Build history of the part. All positions in model axes, mm. A direction names the side the tool comes from. Coordinates: 2 decimals unless noted, no trailing zeros. Write each loop counter-clockwise with the first axis right and the second up, starting at its lowest first coordinate (ties: lowest second). Pieces come first, ordered by that corner, then holes.
```python
from build123d import *

# Parameters (mm, degrees)
SKETCH1_W                       = 149
SKETCH1_H                       = 40
SKETCH1_W_2                     = 6.3
SKETCH1_H_2                     = 6.3
BOSS_EXTRUDE1_DEPTH             = 12.7
TAP_DRILL_FOR_M5X0_8_TAP2_D     = 4.2
TAP_DRILL_FOR_M5X0_8_TAP2_DEPTH = 7
TAP_DRILL_FOR_M5X0_8_TAP2_TIP   = 1.2618073
TAP_DRILL_FOR_M5X0_8_TAP3_D     = 4.2


with BuildPart() as part:
    # Sketch1 → Boss-Extrude1 (new body)
    with BuildSketch(Plane.XY):
        with Locations((0, 20)):
            Rectangle(SKETCH1_W, SKETCH1_H)
        with Locations((35, 20)):
            Rectangle(SKETCH1_W_2, SKETCH1_H_2, mode=Mode.SUBTRACT)
    extrude(amount=BOSS_EXTRUDE1_DEPTH)

    # Tap Drill for M5x0.8 Tap2
    with Locations(Plane(origin=(-60, 0, 6.35), x_dir=(-1, 0, 0), z_dir=(0, -1, 0))):
        with Locations((0, 0), (-60, 0), (-120, 0)):
            Hole(TAP_DRILL_FOR_M5X0_8_TAP2_D / 2, depth=TAP_DRILL_FOR_M5X0_8_TAP2_DEPTH)
            with Locations((0, 0, -(TAP_DRILL_FOR_M5X0_8_TAP2_DEPTH + TAP_DRILL_FOR_M5X0_8_TAP2_TIP / 2))):  # 118° drill point
                Cone(0, TAP_DRILL_FOR_M5X0_8_TAP2_D / 2, TAP_DRILL_FOR_M5X0_8_TAP2_TIP, mode=Mode.SUBTRACT)

    # Tap Drill for M5x0.8 Tap3 (through all)
    with Locations(Plane.XY.offset(12.7)):
        with Locations((-65, 30), (-65, 10), (65, 10), (65, 30)):
            Hole(TAP_DRILL_FOR_M5X0_8_TAP3_D / 2)


solid = part.part
```
1. 3-axis set-ups, long thin cutter, end or side, ignore diameter. For faces 4 (the face through (-74.5, 20, 6)), 5 (the face through (-0.46, 3.55, 8.4)), 6 (the face through (35, 16.85, 6)): which of +Z, -Z, +X, -X, +Y, -Y reach the whole face in a straight line?
Computed values:
face 4: +Z, -Z, -X, +Y, -Y
face 5: -Y
face 6: +Z, -Z
2. Saw through at C-C on z = 11.25. List the corners of the cut face in (x, y).
Computed values:
outline: (-74.5, 0) - (74.5, 0) - (74.5, 40) - (-74.5, 40) - close; hole circle Ø4.2 at (-65, 10); hole circle Ø4.2 at (-65, 30); hole (31.85, 16.85) - (38.15, 16.85) - (38.15, 23.15) - (31.85, 23.15) - close; hole circle Ø4.2 at (65, 10); hole circle Ø4.2 at (65, 30)
3. Saw through at A-A on x = 65. List the corners of the cut face in (y, z).
Computed values:
outline: (0, 0) - (7.9, 0) - (7.9, 12.7) - (0, 12.7) - close; (12.1, 0) - (27.9, 0) - (27.9, 12.7) - (12.1, 12.7) - close; (32.1, 0) - (40, 0) - (40, 12.7) - (32.1, 12.7) - close
4. Probe line 1 along Y through (x, z) = (-65, 3); line 2 along X through (y, z) = (2.5, 6); line 3 along X through (y, z) = (11, 4). List the from-to ranges inside material, lowest first.
Computed values:
line 1: y = 0 to 7.9, 12.1 to 27.9, 32.1 to 40
line 2: x = -74.5 to -62.07, -57.93 to -2.07, 2.07 to 57.93, 62.07 to 74.5
line 3: x = -74.5 to -66.85, -63.15 to 63.15, 66.85 to 74.5
5. Mould opens along Y. For faces 1 (the face through (-60.35, 8.04, 6.24)), 2 (the face through (-1, 20, 0)), 3 (the face through (64.031, 28.137, 6.261)) say: +Y half, -Y half, draft (parallel to the pull), parting line (faces both ways), or undercut.
Computed values:
face 1: -Y half
face 2: draft
face 3: undercut
6. Saw through at B-B on y = 4.5. List the corners of the cut face in (x, z), plus the area to 3 significant figures.
Computed values:
outline: (-74.5, 0) - (74.5, 0) - (74.5, 12.7) - (-74.5, 12.7) - close; hole circle Ø4.2 at (-60, 6.35); hole circle Ø4.2 at (0, 6.35); hole circle Ø4.2 at (60, 6.35)
area: 1,850 mm2
